Can you work these out from the model? Positions are in its coordinate system, mm. A direction names the side the tool comes from. Give positions to 0.01 mm unless a question says otherwise; leave off trailing zeros. Order: outer loops, then holes, each group sorted by start corner. A loop starts at its lowest first (then second) coordinate and runs counter-clockwise, first axis right, second up. Notation, with made-up numbers: M -9,68.25 L -2,68.25 A18 ccw -2,73.25 Z; hole C 71.25,66.25 d10. An arc over 180 degrees is marked long. Answer as a JSON object with one key per item and string values.
```python
from build123d import *

# Parameters (mm, degrees)
ESBO_O1_R                = 4
ESBO_O1_R_2              = 11
RESSALTO_EXTRUS_O1_DEPTH = 8


with BuildPart() as part:
    # Esboço1 → Ressalto-extrusão1 (new body)
    with BuildSketch(Plane(origin=(0, 0, 0), x_dir=(1, 0, 0), z_dir=(0, 1, 0))):
        with BuildLine():
            Line((-33.07179677, 4), (-20.712315177, 4))
            ThreePointArc((-20.712315177, 4), (-16.021899417, 5.168239134), (-12.427389106, 8.4))
            ThreePointArc((-12.427389106, 8.4), (0, 15), (12.427389106, 8.4))
            ThreePointArc((12.427389106, 8.4), (16.021899417, 5.168239134), (20.712315177, 4))
            Line((20.712315177, 4), (33.07179677, 4))
            ThreePointArc((33.07179677, 4), (48, 0), (33.07179677, -4))
            Line((33.07179677, -4), (20.712315177, -4))
            ThreePointArc((20.712315177, -4), (16.021899417, -5.168239134), (12.427389106, -8.4))
            ThreePointArc((12.427389106, -8.4), (0, -15), (-12.427389106, -8.4))
            ThreePointArc((-12.427389106, -8.4), (-16.021899417, -5.168239134), (-20.712315177, -4))
            Line((-20.712315177, -4), (-33.07179677, -4))
            ThreePointArc((-33.07179677, -4), (-48, 0), (-33.07179677, 4))
        make_face()
        with Locations(Location((40, 0, 0), (0, 0, 270))):
            Circle(ESBO_O1_R, mode=Mode.SUBTRACT)
        with Locations(Location((-40, 0, 0), (0, 0, 270))):
            Circle(ESBO_O1_R, mode=Mode.SUBTRACT)
        with Locations(Location((0, 0, 0), (0, 0, 270))):
            Circle(ESBO_O1_R_2, mode=Mode.SUBTRACT)
    extrude(amount=RESSALTO_EXTRUS_O1_DEPTH)


solid = part.part
```
1) For faces 1 (the face through (27, 4, 4)), 2 (the face through (-27, 4, -4)), 3 (the face through (-36.034, 3.944, -0.521)), which set-ups out of +Z, -Z, +X, -X, +Y, -Y let a thin tool reach every point of the face, with its end or its side?
Results found:
{"face 1": "+Z, +Y, -Y", "face 2": "-Z, +Y, -Y", "face 3": "+Y, -Y"}
2) I want a section at C-C on z = 0. Write out the boundary of the cut face in (x, y), and give its area (3 significant figures).
Results found:
{"outline": "M -48,0 L -44,0 L -44,8 L -48,8 Z; M -36,0 L -11,0 L -11,8 L -36,8 Z; M 11,0 L 36,0 L 36,8 L 11,8 Z; M 44,0 L 48,0 L 48,8 L 44,8 Z", "area": "464 mm²"}
3) I need wall thicknesses on L1, parallel to X at y = 3, z = 0; L2, parallel to X at y = 7.5, z = 3.25; L3, parallel to Z at x = -27, y = 6.5. Which ranges of each line are inside material? Lowest first, please.
Results found:
{"L1": "x = -48 to -44, -36 to -11, 11 to 36, 44 to 48", "L2": "x = -47.31 to -42.33, -37.67 to -10.51, 10.51 to 37.67, 42.33 to 47.31", "L3": "z = -4 to 4"}
4) I want a section at B-B on y = 1. Write out the boundary of the cut face in (x, z), and give its area (3 significant figures).
Results found:
{"outline": "M -33.07,-4 L -20.71,-4 A10 cw -12.43,-8.4 A15 ccw 12.43,-8.4 A10 cw 20.71,-4 L 33.07,-4 A8 ccw long 33.07,4 L 20.71,4 A10 cw 12.43,8.4 A15 ccw -12.43,8.4 A10 cw -20.71,4 L -33.07,4 A8 ccw long Z; hole C -40,0 d8; hole C 0,0 d22; hole C 40,0 d8", "area": "932 mm²"}
5) I'm going to push flat-ended pins straight in: pin 1 Ø3 at (x, y) = (-9, 1.5) entering from +Z; pin 2 Ø2.5 at (x, y) = (-24, 2.5) entering from -Z; pin 3 Ø4 at (x, y) = (28.5, 2.5) entering from +Z. Where does each tip first touch, or does it pass through?
Results found:
{"pin 1": "stops at z = 12.99", "pin 2": "stops at z = -4", "pin 3": "stops at z = 4"}
6) I want a section at D-D on x = 27. Write out the boundary of the cut face in (y, z), and give its area (3 significant figures).
Results found:
{"outline": "M 0,-4 L 8,-4 L 8,4 L 0,4 Z", "area": "64.0 mm²"}
7) I want a section at A-A on x = 40. Write out the boundary of the cut face in (y, z), and give its area (3 significant figures).
Results found:
{"outline": "M 0,-8 L 8,-8 L 8,-4 L 0,-4 Z; M 0,4 L 8,4 L 8,8 L 0,8 Z", "area": "64.0 mm²"}
8) Thinking about a two-plate mould opening in Z: for faces 4 (the face through (43.966, 3.944, -0.521)), 5 (the face through (15.96, 3.94, -5.2)), 6 (the face through (-48, 4, 0)), which applies, pulls with the +Z half, pulls with the -Z half, needs draft (parallel to the pull), parting line crosses it, or undercut?
Results found:
{"face 4": "undercut", "face 5": "pulls with the -Z half", "face 6": "parting line crosses it"}
